Could you check a few things on this model? Use its own coordinates, in mm. A direction names the side the tool comes from. Coordinates: 2 decimals unless noted, no trailing zeros. Loops run counter-clockwise (first coordinate to the right, second up) from the corner with the lowest first, then second, coordinate; pieces in that order, holes last.
from build123d import *

# Parameters (mm, degrees)
SKETCH1_R               = 40
SKETCH1_R_2             = 35
BOSS_EXTRUDE1_DEPTH     = 180
BOSS_EXTRUDE2_DEPTH     = 50
SKETCH6_R               = 5.5
BOSS_EXTRUDE3_DEPTH     = 8
CUT_EXTRUDE1_REACH      = 154.121
SKETCH7_R               = 1.55
CUT_EXTRUDE2_START      = -50
SKETCH9_R               = 40
CUT_EXTRUDE2_DEPTH      = 50
CUT_EXTRUDE3_REACH      = 203.684
CUT_EXTRUDE3_END_RADIUS = 30
SKETCH11_R              = 1.5
CIRPATTERN1_COUNT       = 3
CUT_EXTRUDE4_REACH      = 203.684
CUT_EXTRUDE4_END_RADIUS = 35
SKETCH12_R              = 4


with BuildPart() as part:
    # Sketch1 → Boss-Extrude1 (new body)
    with BuildSketch(Plane(origin=(0, 0, 0), x_dir=(1, 0, 0), z_dir=(0, 1, 0))):
        with Locations(Location((0, 0, 0), (0, 0, 90))):
            Circle(SKETCH1_R)
        with Locations(Location((0, 0, 0), (0, 0, 90))):
            Circle(SKETCH1_R_2, mode=Mode.SUBTRACT)
    extrude(amount=BOSS_EXTRUDE1_DEPTH)

    # Sketch3 → Revolve1 (revolve)
    with BuildSketch(Plane(origin=(0, 0, 0), x_dir=(0, 0, -1), z_dir=(1, 0, 0)), mode=Mode.PRIVATE) as revolve1_sk:
        with BuildLine():
            Line((-35, 180), (-40, 180))
            Line((-40, 180), (-40, 185))
            add(Edge.make_bspline(
                [(-20, 210), (-35.448934618, 201.981430701), (-40, 185)],
                knots=[0, 0, 0, 1, 1, 1], degree=2))
            Line((-20, 210), (0, 210))
            Line((0, 210), (0, 202.928932188))
            Line((0, 202.928932188), (-20, 202.928932188))
            add(Edge.make_bspline(
                [(-20, 202.928932188), (-32.989454859, 194.577869332), (-35, 180)],
                knots=[0, 0, 0, 1, 1, 1], degree=2))
        make_face()
    revolve(revolve1_sk.sketch.rotate(Axis((0, -20.154872571, 0), (0, 1, 0)), 180), axis=Axis((0, -20.154872571, 0), (0, 1, 0)))

    # Sketch4 → Boss-Extrude2 (add)
    with BuildSketch(Plane(origin=(0, 0, 0), x_dir=(1, 0, 0), z_dir=(0, 1, 0))):
        with BuildLine():
            Line((4.472135955, 55.245966692), (3.75, 53.995190528))
            ThreePointArc((3.75, 53.995190528), (0, 40), (-3.75, 53.995190528))
            Line((-3.75, 53.995190528), (-4.472135955, 55.245966692))
            ThreePointArc((-4.472135955, 55.245966692), (-5.133489086, 55.72479725), (-5.931290399, 55.551074103))
            ThreePointArc((-5.931290399, 55.551074103), (-9.440614698, 50.797695275), (-9.654223492, 44.893092105))
            ThreePointArc((-9.654223492, 44.893092105), (-10.13118194, 40.546025245), (-13.431963119, 37.677345538))
            Line((-13.431963119, 37.677345538), (13.431963119, 37.677345538))
            ThreePointArc((13.431963119, 37.677345538), (10.13118194, 40.546025245), (9.654223492, 44.893092105))
            ThreePointArc((9.654223492, 44.893092105), (9.440614698, 50.797695275), (5.931290399, 55.551074103))
            ThreePointArc((5.931290399, 55.551074103), (5.133489086, 55.72479725), (4.472135955, 55.245966692))
        make_face()
        with BuildLine():
            Line((45.608342635, -31.495966692), (44.88620668, -30.245190528))
            ThreePointArc((44.88620668, -30.245190528), (34.641016151, -20), (48.63620668, -23.75))
            Line((48.63620668, -23.75), (50.08047859, -23.75))
            ThreePointArc((50.08047859, -23.75), (50.825834582, -23.416666667), (51.07428658, -22.638888889))
            ThreePointArc((51.07428658, -22.638888889), (48.712401911, -17.223035482), (43.705669963, -14.085743255))
            ThreePointArc((43.705669963, -14.085743255), (40.179478855, -11.499151692), (39.345519942, -7.206251485))
            Line((39.345519942, -7.206251485), (25.913556823, -30.471094053))
            ThreePointArc((25.913556823, -30.471094053), (30.048296914, -29.046873553), (34.051446472, -30.80734885))
            ThreePointArc((34.051446472, -30.80734885), (39.271787213, -33.574659793), (45.142996181, -32.912185214))
            ThreePointArc((45.142996181, -32.912185214), (45.692345496, -32.308130583), (45.608342635, -31.495966692))
        make_face()
        with BuildLine():
            Line((-50.08047859, -23.75), (-48.63620668, -23.75))
            ThreePointArc((-48.63620668, -23.75), (-34.641016151, -20), (-44.88620668, -30.245190528))
            Line((-44.88620668, -30.245190528), (-45.608342635, -31.495966692))
            ThreePointArc((-45.608342635, -31.495966692), (-45.692345496, -32.308130583), (-45.142996181, -32.912185214))
            ThreePointArc((-45.142996181, -32.912185214), (-39.271787213, -33.574659793), (-34.051446472, -30.80734885))
            ThreePointArc((-34.051446472, -30.80734885), (-30.048296914, -29.046873553), (-25.913556823, -30.471094053))
            Line((-25.913556823, -30.471094053), (-39.345519942, -7.206251485))
            ThreePointArc((-39.345519942, -7.206251485), (-40.179478855, -11.499151692), (-43.705669963, -14.085743255))
            ThreePointArc((-43.705669963, -14.085743255), (-48.712401911, -17.223035482), (-51.07428658, -22.638888889))
            ThreePointArc((-51.07428658, -22.638888889), (-50.825834582, -23.416666667), (-50.08047859, -23.75))
        make_face()
    extrude(amount=BOSS_EXTRUDE2_DEPTH)

    # Sketch6 → Boss-Extrude3 (add)
    with BuildSketch(Plane(origin=(0, 70, 0), x_dir=(1, 0, 0), z_dir=(0, 1, 0))):
        with BuildLine():
            Line((-5, 34.641016151), (-5, 11.456439237))
            ThreePointArc((-5, 11.456439237), (-10.458250332, 6.846531969), (-12.5, 0))
            Line((-12.5, 0), (-32.948700726, -11.806062869))
            ThreePointArc((-32.948700726, -11.806062869), (-30.310889132, -17.5), (-26.698700726, -22.631380416))
            Line((-26.698700726, -22.631380416), (-6.25, -10.825317547))
            ThreePointArc((-6.25, -10.825317547), (0, -12.5), (6.25, -10.825317547))
            Line((6.25, -10.825317547), (26.698700726, -22.631380416))
            ThreePointArc((26.698700726, -22.631380416), (30.310889132, -17.5), (32.948700726, -11.806062869))
            Line((32.948700726, -11.806062869), (12.5, 0))
            ThreePointArc((12.5, 0), (10.458250332, 6.846531969), (5, 11.456439237))
            Line((5, 11.456439237), (5, 34.641016151))
            ThreePointArc((5, 34.641016151), (0, 35), (-5, 34.641016151))
        make_face()
        with Locations(Location((0, 0, 0), (0, 0, 270))):
            Circle(SKETCH6_R, mode=Mode.SUBTRACT)
    extrude(amount=BOSS_EXTRUDE3_DEPTH)

    # Sketch7 → Cut-Extrude1 (cut, up to next)
    with BuildSketch(Plane(origin=(0, 78, 0), x_dir=(1, 0, 0), z_dir=(0, 1, 0)), mode=Mode.PRIVATE) as cut_extrude1_sk1:
        with Locations(Location((0, 8, 0), (0, 0, 270))):
            Circle(SKETCH7_R)
    cut_extrude1_tool1 = extrude(cut_extrude1_sk1.sketch, amount=-CUT_EXTRUDE1_REACH, mode=Mode.PRIVATE) & part.part
    # Sketch7 → Cut-Extrude1 (cut, up to next)
    with BuildSketch(Plane(origin=(0, 78, 0), x_dir=(1, 0, 0), z_dir=(0, 1, 0)), mode=Mode.PRIVATE) as cut_extrude1_sk2:
        with Locations(Location((8, 0, 0), (0, 0, 270))):
            Circle(SKETCH7_R)
    cut_extrude1_tool2 = extrude(cut_extrude1_sk2.sketch, amount=-CUT_EXTRUDE1_REACH, mode=Mode.PRIVATE) & part.part
    # Sketch7 → Cut-Extrude1 (cut, up to next)
    with BuildSketch(Plane(origin=(0, 78, 0), x_dir=(1, 0, 0), z_dir=(0, 1, 0)), mode=Mode.PRIVATE) as cut_extrude1_sk3:
        with Locations(Location((0, -8, 0), (0, 0, 270))):
            Circle(SKETCH7_R)
    cut_extrude1_tool3 = extrude(cut_extrude1_sk3.sketch, amount=-CUT_EXTRUDE1_REACH, mode=Mode.PRIVATE) & part.part
    # Sketch7 → Cut-Extrude1 (cut, up to next)
    with BuildSketch(Plane(origin=(0, 78, 0), x_dir=(1, 0, 0), z_dir=(0, 1, 0)), mode=Mode.PRIVATE) as cut_extrude1_sk4:
        with Locations(Location((-8, 0, 0), (0, 0, 270))):
            Circle(SKETCH7_R)
    cut_extrude1_tool4 = extrude(cut_extrude1_sk4.sketch, amount=-CUT_EXTRUDE1_REACH, mode=Mode.PRIVATE) & part.part
    add(cut_extrude1_tool1.solids().sort_by_distance((0, 78, -8))[0], mode=Mode.SUBTRACT)
    add(cut_extrude1_tool2.solids().sort_by_distance((8, 78, 0))[0], mode=Mode.SUBTRACT)
    add(cut_extrude1_tool3.solids().sort_by_distance((0, 78, 8))[0], mode=Mode.SUBTRACT)
    add(cut_extrude1_tool4.solids().sort_by_distance((-8, 78, 0))[0], mode=Mode.SUBTRACT)

    # Sketch9 → Cut-Extrude2 (cut)
    with BuildSketch(Plane(origin=(0, 210, 0), x_dir=(1, 0, 0), z_dir=(0, 1, 0)).offset(CUT_EXTRUDE2_START)):
        with Locations(Location((0, 0, 0), (0, 0, 90))):
            Circle(SKETCH9_R)
    extrude(amount=CUT_EXTRUDE2_DEPTH, mode=Mode.SUBTRACT)

    # Sketch10 → Revolve2 (revolve)
    with BuildSketch(Plane.XY, mode=Mode.PRIVATE) as revolve2_sk:
        Polygon((-35, 146.339745962), (-30, 155), (-30, 170), (-34.85, 170), (-34.85, 160), (-35, 160), align=None)
    revolve(revolve2_sk.sketch.rotate(Axis((0, 0, 0), (0, 1, 0)), 270), axis=Axis((0, 0, 0), (0, 1, 0)))

    # Cut-Extrude3: up to this cylinder (the profile starts outside it)
    cut_extrude3_end = Plane(origin=(0, 165, 0), z_dir=(0, -1, 0)) * Cylinder(CUT_EXTRUDE3_END_RADIUS, 468.368, mode=Mode.PRIVATE)
    # Sketch11 → Cut-Extrude3 (cut, up to the surface)
    with BuildSketch(Plane.XY.offset(40), mode=Mode.PRIVATE) as cut_extrude3_sk1:
        with Locations((0, 165)):
            Circle(SKETCH11_R)
    cut_extrude3_tool1 = extrude(cut_extrude3_sk1.sketch, amount=-CUT_EXTRUDE3_REACH, mode=Mode.PRIVATE) - cut_extrude3_end
    cut_extrude3 = cut_extrude3_tool1.solids().sort_by_distance((0, 165, 40))[0]
    add(cut_extrude3, mode=Mode.SUBTRACT)

    # CirPattern1: Cut-Extrude3 ×3 about axis
    cirpattern1_axis = Axis((0, 170, 0), (0, -1, 0))
    for i in range(1, CIRPATTERN1_COUNT):
        add(cut_extrude3.rotate(cirpattern1_axis, i * 360 / CIRPATTERN1_COUNT), mode=Mode.SUBTRACT)

    # Cut-Extrude4: up to this cylinder (the profile starts outside it)
    cut_extrude4_end = Plane(origin=(0, 21.8133005, 0), z_dir=(0, -1, 0)) * Cylinder(CUT_EXTRUDE4_END_RADIUS, 514.741399, mode=Mode.PRIVATE)
    # Sketch12 → Cut-Extrude4 (cut, up to the surface)
    with BuildSketch(Plane.XY.offset(40), mode=Mode.PRIVATE) as cut_extrude4_sk1:
        with Locations((0, 40)):
            Circle(SKETCH12_R)
    cut_extrude4_tool1 = extrude(cut_extrude4_sk1.sketch, amount=-CUT_EXTRUDE4_REACH, mode=Mode.PRIVATE) - cut_extrude4_end
    add(cut_extrude4_tool1.solids().sort_by_distance((0, 40, 40))[0], mode=Mode.SUBTRACT)
    # Sketch12 → Cut-Extrude4 (cut, up to the surface)
    with BuildSketch(Plane.XY.offset(40), mode=Mode.PRIVATE) as cut_extrude4_sk2:
        with BuildLine():
            Line((-4, 0), (4, 0))
            Line((4, 0), (4, 4))
            ThreePointArc((4, 4), (0, 8), (-4, 4))
            Line((-4, 4), (-4, 0))
        make_face()
    cut_extrude4_tool2 = extrude(cut_extrude4_sk2.sketch, amount=-CUT_EXTRUDE4_REACH, mode=Mode.PRIVATE) - cut_extrude4_end
    add(cut_extrude4_tool2.solids().sort_by_distance((0, 3.626601, 40))[0], mode=Mode.SUBTRACT)


solid = part.part
(1) We'd pull the mould along X, two halves only. Please class faces 6 (the face through (0, 8, 37)), 7 (the face through (-34.3, 0, -8.2)), 8 (the face through (40.21, 24.65, 11.55)): +X half, -X half, draft (parallel to the pull), parting line (faces both ways), or undercut.
Answers:
face 6: undercut
face 7: draft
face 8: +X half
(2) Imagine slicing it at C-C, the plane z = -27. State how many separate pieces and enclosed holes the cut face has, and give its area (3 significant figures).
Answers:
separate pieces: 3
enclosed holes: 0
area: 2,740 mm2
(3) I need wall thicknesses on probe 1 along Z at (x, y) = (0, 31); probe 2 along X at (y, z) = (27, 23); probe 3 along Z at (x, y) = (29, 68). Which ranges of each line are inside material? Lowest first, please.
Answers:
probe 1: z = -40 to -35, 35 to 40
probe 2: x = -51.05 to -48.6, -33.67 to -26.38, 26.38 to 33.67, 48.6 to 51.05
probe 3: z = -27.55 to -19.6, 19.6 to 27.55
(4) Which directions (+Z, -Z, +X, -X, +Y, -Y) give clear straight access to the entire face, cutting with the end or side of a thin tool? Please do faces 1 (the face through (-12.015, 78.88, -38.153)), 2 (the face through (10.16, 24.65, -40.49)), 3 (the face through (43, 50, 16)), 4 (the face through (5, 70, 6)), 5 (the face through (4, 2, 37)).
Answers:
face 1: +Y
face 2: +X, +Y, -Y
face 3: +Z, +X, +Y
face 4: -Y
face 5: +Z, -Y
(5) For pin 1 (3 mm diameter, centred on x = 8, z = 0, fed in from -Y); pin 2 (3 mm diameter, centred on y = 2.5, z = 38.5, fed in from -X); pin 3 (4 mm diameter, centred on y = 72.5, z = -25, fed in from -X); pin 4 (5 mm diameter, centred on x = 21, y = 55, fed in from -Z), each with a flat end and sliding along its axis, tell me the tip position at first contact or that it passes through.
Answers:
pin 1: passes through
pin 2: stops at x = -15.2
pin 3: stops at x = -32.73
pin 4: stops at z = -35.46
(6) Imagine slicing it at B-B, the plane y = 136. Write out the boundary of the cut face in (x, z).
Answers:
outline: circle Ø80 at (0, 0); hole circle Ø70 at (0, 0)
